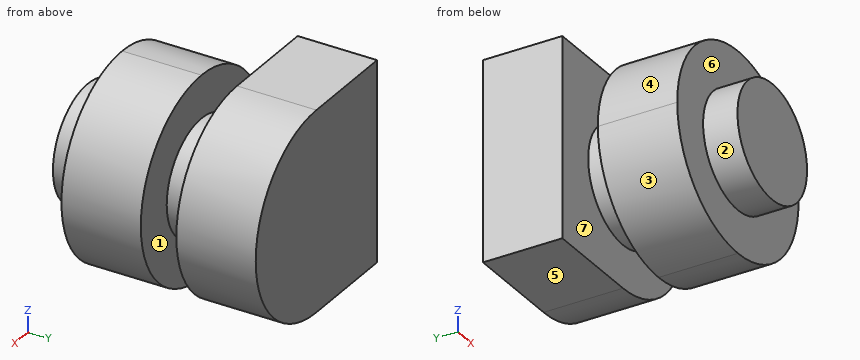
Autodesk Inventor part; units mm, degrees
ref_plane "XZ Plane" through (0, 0, 0) normal (0, 1, 0) x (-1, 0, 0)
ref_plane "XY Plane" through (0, 0, 0) normal (0, 0, 1) x (1, 0, 0)
sketch "Sketch1" plane through (0, 0, 0) normal (0, 1, 0) x (-1, 0, 0)
  line L0 (13.075, -26.15) -> (-13.075, -26.15)
  line L1 (-13.075, -26.15) -> (-13.075, 26.15)
  line L2 (-13.075, 26.15) -> (13.075, 26.15)
  line L3 (13.075, 26.15) -> (13.075, -26.15)
  arc A0 (-13.075, 26.15) -> (-13.075, -26.15) centre (-13.075, 0) ccw
  circle A1 centre (-13.075, 0) radius 26.15
  point P0 (0, 0)
  point P1 (0, -26.15)
  dimension "d0" = 26.15
extrude "Extrusion1" add sketch "Sketch1" along normal blind 20.8
sketch "Sketch2" plane through (0, 20.8, 0) normal (0, 1, 0) x (1, 0, 0)
  circle A0 centre (13.075, 0) radius 15
  arc A1 (13.075, -26.15) -> (13.075, 26.15) centre (13.075, 0) ccw
  point P0 (0, 0)
  dimension "d3" = 30
extrude "Extrusion2" add sketch "Sketch2" along normal blind 9.3
sketch "Sketch3" plane through (0, 0, 0) normal (0, -1, 0) x (1, 0, 0)
  circle A0 centre (13.075, 0) radius 15
  arc A1 (13.075, -26.15) -> (13.075, 26.15) centre (13.075, 0) ccw
  point P0 (0, 0)
  dimension "d6" = 30
extrude "Extrusion3" add sketch "Sketch3" along normal blind 9
sketch "Sketch4" plane through (13.075, 30.1, 0) normal (0, 1, 0) x (1, 0, 0)
  line L0 (-26.15, 26.15) -> (-26.15, -26.15)
  line L1 (-26.15, -26.15) -> (-26.15, 26.15)
  line L2 (0, 26.15) -> (-26.15, 26.15)
  line L3 (-26.15, 26.15) -> (0, 26.15)
  arc A0 (0, -26.15) -> (0, 26.15) centre (0, 0) ccw
  arc A1 (0, -26.15) -> (0, 26.15) centre (0, 0) ccw
  line L4 (-26.15, -26.15) -> (0, -26.15)
  line L5 (0, -26.15) -> (-26.15, -26.15)
  point P0 (-13.075, 0)
extrude "Extrusion4" add sketch "Sketch4" along normal blind 20.8
fillet "Fillet1" radius 26.15 2 edges at (-13.075, 10.4, -26.15) (-13.075, 10.4, 26.15)
properties part number "Table Hinge"
For this review, take the finished solid that the model builds, in its own axes (mm). Face numbers are marked on the shaded views. A direction names the side the tool comes from. Give positions to 0.01 mm unless a question says otherwise; leave off trailing zeros. Loops run counter-clockwise (first coordinate to the right, second up) from the corner with the lowest first, then second, coordinate; pieces in that order, holes last. Notation, with made-up numbers: M 62,48 L 102,48 A12 ccw 102,52 Z; hole C -17,25 d5. An arc over 180 degrees is marked long. One line per item, written item: value. Start each with the question number.
Q1. Add section D-D (x = 17.5). Give the boundary of the cut face in (y, z).
Q2. For L1, parallel to Y at x = -0.5, z = -11; L2, parallel to Z at x = 13.5, y = 35; L3, parallel to X at y = 30, z = 0.5, list the stretches that pass through material, from the lowest coordinate up.
Q3. Add section A-A (x = -6.5). Give the boundary of the cut face in (y, z).
Q4. Clearance check with flat-ended pins moving along their axes: pin 1 Ø1.5 at (x, z) = (30, -9.5) entering from -Y; pin 2 Ø8 at (x, z) = (18, -17) entering from -Y; pin 3 Ø1.5 at (y, z) = (32.5, -9.5) entering from +X; pin 4 Ø1 at (x, y) = (15, 28.5) entering from -Z. State where each tip first meets the part, or that it passes through.
Q5. Add section C-C (z = -9.5). Give the boundary of the cut face in (x, y) (3 decimals).
Q6. Draft analysis for pull direction Y (two halves, no side actions). For the marked faces 5, 6 and 7, state which applies: released by +Y, released by -Y, zero draft, split by the parting line, or undercut.
Q7. Machinability: for the marked faces 1, 2, 3 and 4, which of the approach directions +Z, -Z, +X, -X, +Y, -Y give a long, thin tool a straight path to every point of the face, cutting with its end or side? Answer none if there is none.
Reply:
1. outline: M -9,-14.33 L 0,-14.33 L 0,-25.77 L 20.8,-25.77 L 20.8,-14.33 L 30.1,-14.33 L 30.1,-25.77 L 50.9,-25.77 L 50.9,25.77 L 30.1,25.77 L 30.1,14.33 L 20.8,14.33 L 20.8,25.77 L 0,25.77 L 0,14.33 L -9,14.33 Z
2. L1: 0 to 20.8, 30.1 to 50.9
2. L2: -26.15 to 26.15
2. L3: -1.92 to 28.07
3. outline: M 0,-17.34 L 20.8,-17.34 L 20.8,17.34 L 0,17.34 Z; M 30.1,-26.15 L 50.9,-26.15 L 50.9,26.15 L 30.1,26.15 Z
4. pin 1: y = 0
4. pin 2: y = -9
4. pin 3: x = 37.72
4. pin 4: z = -14.93
5. outline: M -13.075,30.1 L 1.467,30.1 L 1.467,20.8 L -11.288,20.8 L -11.288,0 L 1.467,0 L 1.467,-9 L 24.683,-9 L 24.683,0 L 37.438,0 L 37.438,20.8 L 24.683,20.8 L 24.683,30.1 L 37.438,30.1 L 37.438,50.9 L -13.075,50.9 Z
6. face 5: zero draft
6. face 6: released by -Y
6. face 7: undercut
7. face 1: none
7. face 2: -Y
7. face 3: -Z, -X, -Y
7. face 4: +Z, -X, -Y
